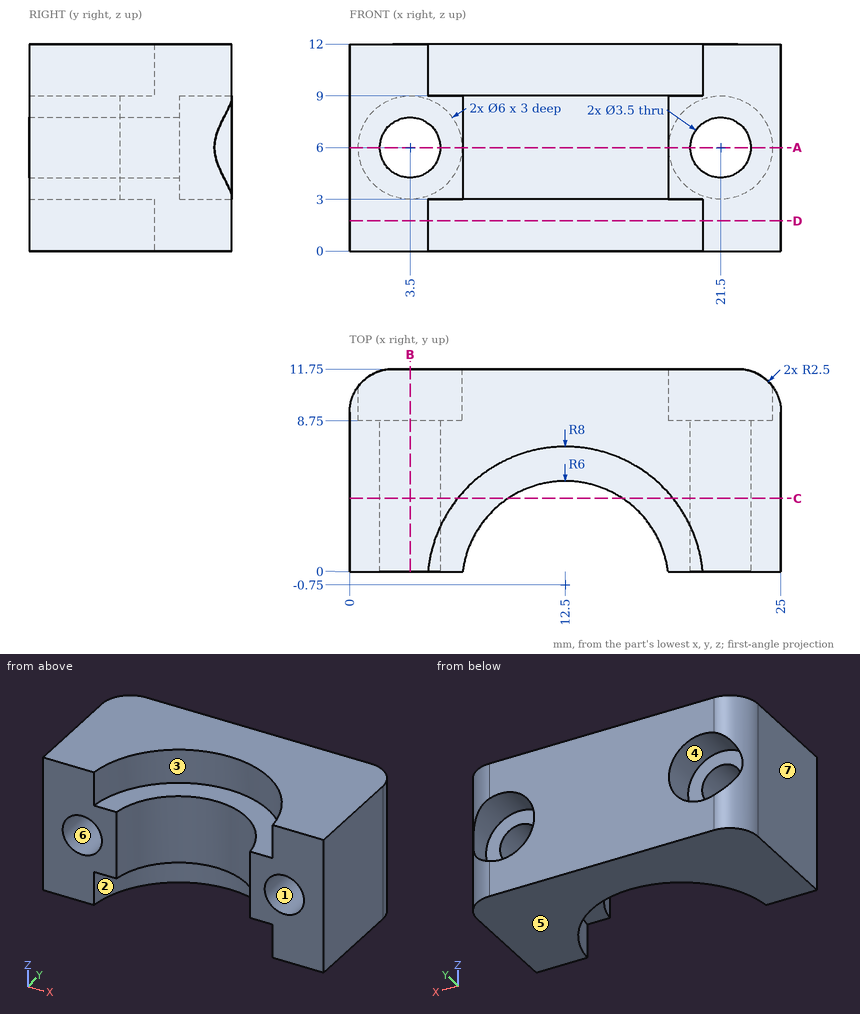
Design review of the part shown in the three views and the two pictorial views. Dimensions are in mm from the part's minimum x, y and z. A direction names the side the tool comes from. Give positions to 0.01 mm unless a question says otherwise; leave off trailing zeros. Loops run counter-clockwise (first coordinate to the right, second up) from the corner with the lowest first, then second, coordinate; pieces in that order, holes last. Notation, with made-up numbers: (25.5, 75.5) -> (84.5, 75.5) arc R21 cw to (84.5, 97.5) -> close; hole circle Ø2 at (-19.75, 71). An arc over 180 degrees is marked (long way). Write each question's results on one line, items separated by ' | '.
1) Take a section at B-B, the plane x = 3.5. Give the boundary of the cut face in (y, z).
Conclusion:
outline: (0, 0) -> (11.75, 0) -> (11.75, 3) -> (8.75, 3) -> (8.75, 4.25) -> (0, 4.25) -> close; (0, 7.75) -> (8.75, 7.75) -> (8.75, 9) -> (11.75, 9) -> (11.75, 12) -> (0, 12) -> close
2) Take a section at C-C, the plane y = 4.25. Give the boundary of the cut face in (x, z) (3 decimals), plus the area to 3 significant figures.
Conclusion:
outline: (0, 0) -> (6.255, 0) -> (6.255, 3) -> (9.183, 3) -> (9.183, 9) -> (6.255, 9) -> (6.255, 12) -> (0, 12) -> close; (15.817, 3) -> (18.745, 3) -> (18.745, 0) -> (25, 0) -> (25, 12) -> (18.745, 12) -> (18.745, 9) -> (15.817, 9) -> close; hole circle Ø3.5 at (3.5, 6); hole circle Ø3.5 at (21.5, 6) | area: 166 mm^2
3) Tool access review of the marked faces 1, 2, 3 and 4: name each direction out of +Z, -Z, +X, -X, +Y, -Y from which nothing blocks a thin tool from reaching the whole face with its end or side.
Conclusion:
face 1: +Y, -Y | face 2: -Z, -Y | face 3: +Z, -Y | face 4: +Y
4) Take a section at A-A, the plane z = 6. Give the boundary of the cut face in (x, y).
Conclusion:
outline: (0, 0) -> (1.75, 0) -> (1.75, 8.75) -> (0.5, 8.75) -> (0.5, 10.75) arc R2.5 ccw to (0, 9.25) -> close; (5.25, 0) -> (6.55, 0) arc R6 cw to (18.45, 0) -> (19.75, 0) -> (19.75, 8.75) -> (18.5, 8.75) -> (18.5, 11.75) -> (6.5, 11.75) -> (6.5, 8.75) -> (5.25, 8.75) -> close; (23.25, 0) -> (25, 0) -> (25, 9.25) arc R2.5 ccw to (24.5, 10.75) -> (24.5, 8.75) -> (23.25, 8.75) -> close
5) Take a section at D-D, the plane z = 1.75. Give the boundary of the cut face in (x, y).
Conclusion:
outline: (0, 0) -> (4.54, 0) arc R8 cw to (20.46, 0) -> (25, 0) -> (25, 9.25) arc R2.5 ccw to (22.5, 11.75) -> (2.5, 11.75) arc R2.5 ccw to (0, 9.25) -> close
6) Insertion check: pin 1 Ø2 at (x, y) = (13.5, 3.5) entering from -Z; pin 2 Ø1 at (x, z) = (2.5, 7) entering from +Y; pin 3 Ø3.5 at (x, y) = (9, 2) entering from -Z. Each pin has a flat end and moves straight along its axis. Give the tip position at first contact, or say it passes through.
Conclusion:
pin 1: passes through | pin 2: stops at y = 8.75 | pin 3: stops at z = 3
7) For line 1 along Z through (x, y) = (3.5, 10.1); line 2 along X through (y, z) = (2, 4.75); line 3 along X through (y, z) = (4, 4.5), list the stretches that pass through material, from the lowest coordinate up. Write a range as from..to.
Conclusion:
line 1: z = 0..3, 9..12 | line 2: x = 0..2.28, 4.72..7.17, 17.83..20.28, 22.72..25 | line 3: x = 0..2.6, 4.4..8.83, 16.17..20.6, 22.4..25
8) Draft analysis for pull direction Z (two halves, no side actions). For the marked faces 5, 6 and 7, state which applies: pulls with the +Z half, pulls with the -Z half, needs draft (parallel to the pull), parting line crosses it, or undercut.
Conclusion:
face 5: pulls with the -Z half | face 6: undercut | face 7: needs draft
